Input: dimensioned drawing with shaded views. Units: mm. Origin: part minimum x, y, z. A direction names the side the tool comes from. Coordinates: 2 decimals unless noted, no trailing zeros. Loops run counter-clockwise (first coordinate to the right, second up) from the corner with the lowest first, then second, coordinate; pieces in that order, holes last. Notation, with made-up numbers: (58, 70.5) -> (72, 70.5) arc R17 ccw to (72, 82.5) -> close; hole circle Ø9 at (-8.5, 89.5). An arc over 180 degrees is marked (long way). Answer as CSV lines item,"result".
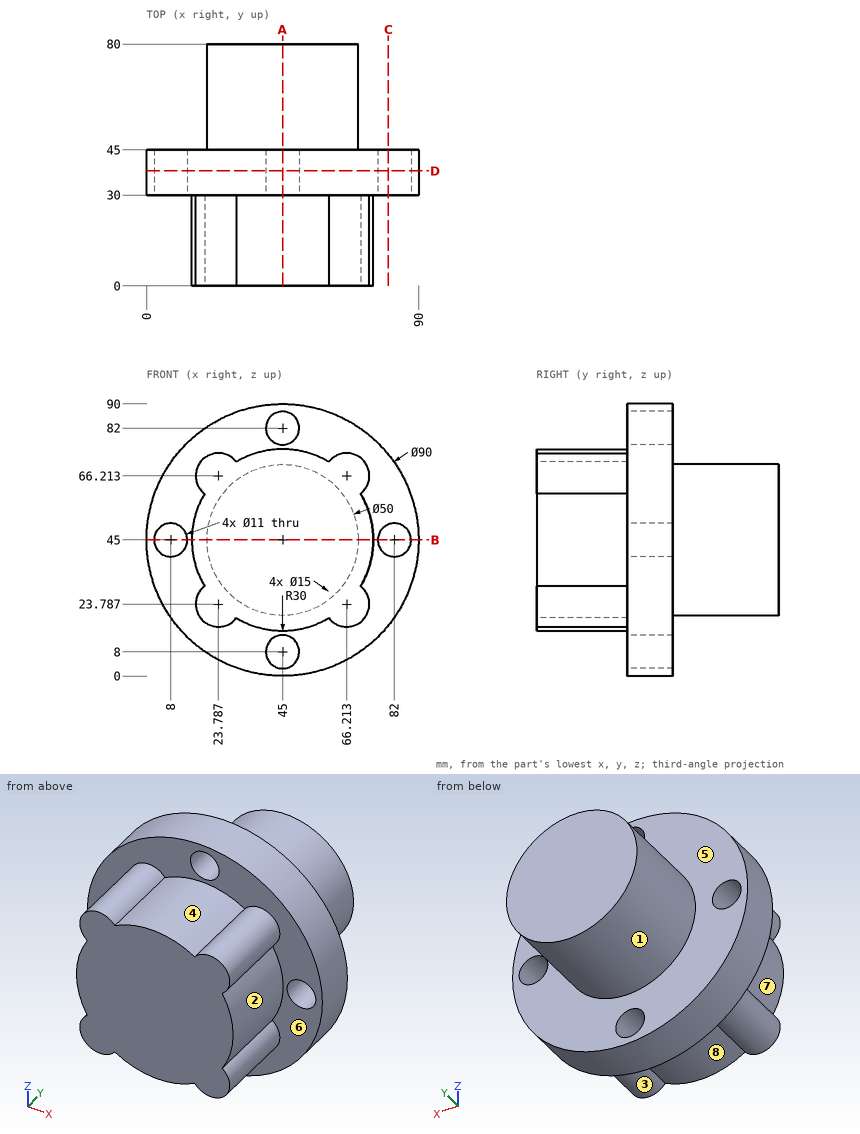
(1) Material intervals for L1, parallel to Z at x = 45, y = 34; L2, parallel to Z at x = 48, y = 37; L3, parallel to X at y = 40.5, z = 8, sorted ascending. Write a range as [from, to].
Computed values:
L1,"[0, 2.5], [13.5, 76.5], [87.5, 90]"
L2,"[0.1, 3.39], [12.61, 77.39], [86.61, 89.9]"
L3,"[19.39, 39.5], [50.5, 70.61]"
(2) Cut plane C-C (x = 80). Return the cut outline in (y, z), then the cut area to 3 significant figures.
Computed values:
outline,"(30, 16.72) -> (45, 16.72) -> (45, 39.88) -> (30, 39.88) -> close; (30, 50.12) -> (45, 50.12) -> (45, 73.28) -> (30, 73.28) -> close"
area,"695 mm^2"
(3) Cut plane D-D (y = 38). Return the cut outline in (x, z).
Computed values:
outline,"circle Ø90 at (45, 45); hole circle Ø11 at (8, 45); hole circle Ø11 at (45, 8); hole circle Ø11 at (45, 82); hole circle Ø11 at (82, 45)"
(4) Draft query along X for the marked faces 1, 2 and 3. Return one class per face: released by +X, released by -X, zero draft, split by the parting line, or undercut.
Computed values:
face 1,"split by the parting line"
face 2,"released by +X"
face 3,"undercut"
(5) Cut plane B-B (z = 45). Return the cut outline in (x, y), then the cut area to 3 significant figures.
Computed values:
outline,"(0, 30) -> (2.5, 30) -> (2.5, 45) -> (0, 45) -> close; (13.5, 30) -> (15, 30) -> (15, 0) -> (75, 0) -> (75, 30) -> (76.5, 30) -> (76.5, 45) -> (70, 45) -> (70, 80) -> (20, 80) -> (20, 45) -> (13.5, 45) -> close; (87.5, 30) -> (90, 30) -> (90, 45) -> (87.5, 45) -> close"
area,"4,570 mm^2"
(6) Access query for the marked faces 4, 5, 6, 7 and 8. Directions: +Z, -Z, +X, -X, +Y, -Y. A direction counts if a zero-diameter tool reaches every point of the face in a straight line with its end or side. Return the directions, or none.
Computed values:
face 4,"+Z, -Y"
face 5,"+Y"
face 6,"-Y"
face 7,"-X, -Y"
face 8,"-Z, -Y"
(7) Cut plane A-A (x = 45). Return the cut outline in (y, z).
Computed values:
outline,"(0, 15) -> (30, 15) -> (30, 13.5) -> (45, 13.5) -> (45, 20) -> (80, 20) -> (80, 70) -> (45, 70) -> (45, 76.5) -> (30, 76.5) -> (30, 75) -> (0, 75) -> close; (30, 0) -> (45, 0) -> (45, 2.5) -> (30, 2.5) -> close; (30, 87.5) -> (45, 87.5) -> (45, 90) -> (30, 90) -> close"
(8) Pin query (flat end, axial travel): pin 1 Ø10 at (x, y) = (63, 60.5) entering from -Z; pin 2 Ø8 at (y, z) = (45.5, 59) entering from -X; pin 3 Ø12 at (x, z) = (10, 63.5) entering from +Y. Return the tip coordinate at first contact, or that it passes through.
Computed values:
pin 1,"z = 23.65"
pin 2,"x = 1.13"
pin 3,"y = 45"
